Study the drawing (mm; zero at the part's minimum x, y, z) and answer. Give positions to 0.01 mm unless a question says otherwise; leave off trailing zeros. Write each loop counter-clockwise with the first axis right and the second up, starting at its lowest first coordinate (ties: lowest second). Pieces come first, ordered by that corner, then holes. Notation, with made-up numbers: (31.25, -25.75) - (69.25, -25.75) arc R10 ccw to (69.25, -11.75) - close; hole circle Ø8 at (-31, -34). An arc over 180 degrees is marked (long way). Write each question's results on one line, items separated by ' | '. Start each with the question number.
Q1. Flat-ended cylindrical pins translate along their axes: pin 1 Ø2 at (y, z) = (8, 15) entering from +X; pin 2 Ø6 at (x, z) = (14.5, 9.5) entering from -Y; pin 3 Ø2 at (y, z) = (7.5, 14) entering from -X; pin 4 Ø2.5 at (x, y) = (9.5, 9.5) entering from +Z. Find the tip coordinate at first contact, or state that the pin passes through.
Q2. Find the intervals of material crossed by probe 1 along Y at (x, z) = (9.5, 10.25); probe 2 along X at (y, z) = (8.75, 4.5); probe 3 along X at (y, z) = (3.25, 12.75), in increasing order.
Q3. Section B-B (z = 4.75) is taken. Determine the outline of the cut face in (x, y), plus the area to 3 significant figures.
Q4. Section A-A (x = 9.5) is taken. Determine the outline of the cut face in (y, z).
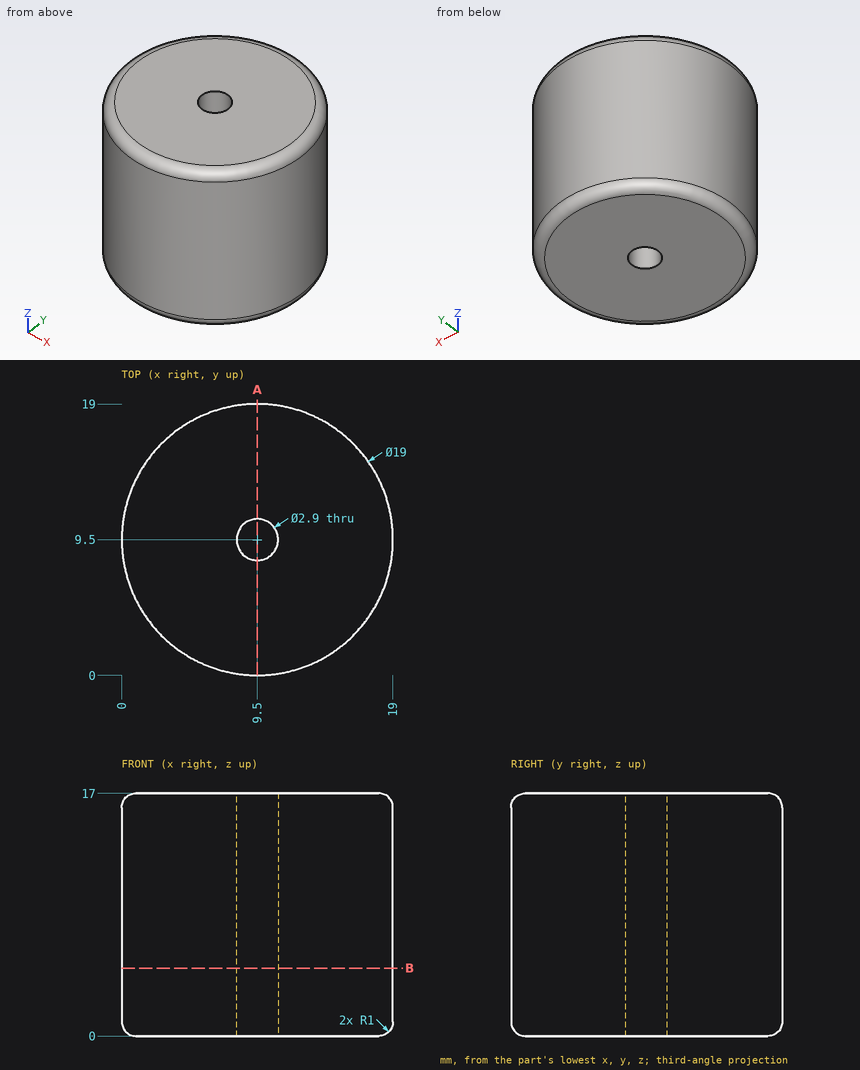
Answers below:
1) pin 1: stops at x = 18.99 | pin 2: stops at y = 0.21 | pin 3: stops at x = 0.05 | pin 4: passes through
2) probe 1: y = 0 to 8.05, 10.95 to 19 | probe 2: x = 0.03 to 8.26, 10.74 to 18.97 | probe 3: x = 2.35 to 16.65
3) outline: circle Ø19 at (9.5, 9.5); hole circle Ø2.9 at (9.5, 9.5) | area: 277 mm2
4) outline: (0, 1) arc R1 ccw to (1, 0) - (8.05, 0) - (8.05, 17) - (1, 17) arc R1 ccw to (0, 16) - close; (10.95, 0) - (18, 0) arc R1 ccw to (19, 1) - (19, 16) arc R1 ccw to (18, 17) - (10.95, 17) - close
